from build123d import *

# Parameters (mm, degrees)
SKETCH1_R           = 22.5
BOSS_EXTRUDE1_DEPTH = 89
SKETCH2_R           = 21
BOSS_EXTRUDE2_DEPTH = 20
SKETCH3_R           = 16
BOSS_EXTRUDE3_DEPTH = 20
CHAMFER1_SIZE       = 5
SKETCH4_R           = 5
BOSS_EXTRUDE4_DEPTH = 13
SKETCH5_R           = 3
CUT_EXTRUDE1_DEPTH  = 10


with BuildPart() as part:
    # Sketch1 → Boss-Extrude1 (new body)
    with BuildSketch(Plane.XY):
        Circle(SKETCH1_R)
    extrude(amount=BOSS_EXTRUDE1_DEPTH)

    # Sketch2 → Boss-Extrude2 (add)
    with BuildSketch(Plane.XY.offset(89)):
        Circle(SKETCH2_R)
    extrude(amount=BOSS_EXTRUDE2_DEPTH)

    # Sketch3 → Boss-Extrude3 (add)
    with BuildSketch(Plane.XY.offset(109)):
        Circle(SKETCH3_R)
    extrude(amount=BOSS_EXTRUDE3_DEPTH)

    # Chamfer1
    chamfer1_edges = [part.edges().sort_by_distance(p)[0] for p in [
        (-16, 0, 129),
    ]]
    chamfer(chamfer1_edges, length=CHAMFER1_SIZE)

    # Sketch4 → Boss-Extrude4 (add)
    with BuildSketch(Plane.XY.offset(129)):
        with Locations(Location((0, 0, 0), (0, 0, 180))):
            Circle(SKETCH4_R)
    extrude(amount=BOSS_EXTRUDE4_DEPTH)

    # Sketch5 → Cut-Extrude1 (cut)
    with BuildSketch(Plane.XY.offset(142)):
        Circle(SKETCH5_R)
    extrude(amount=-CUT_EXTRUDE1_DEPTH, mode=Mode.SUBTRACT)


solid = part.part
The listing builds one solid part. Answer for the finished solid, in the listing's coordinates (mm). A direction names the side the tool comes from. Coordinates: 2 decimals unless noted, no trailing zeros. Order: outer loops, then holes, each group sorted by start corner. A loop starts at its lowest first (then second) coordinate and runs counter-clockwise, first axis right, second up.
Q1. For a pull along Y with two mould halves and no side action, classify faces 3 (the face through (-3, 0, 137)), 4 (the face through (0.1, 3.3, 142)), 5 (the face through (-8.9, -6.8, 128.8)) as pulls with the +Y half, pulls with the -Y half, needs draft (parallel to the pull), parting line crosses it, or undercut.
Q2. Given P1, Ø5, axis at x = 0.5, y = 10.5, coming from the +Z side; P2, Ø3, axis at x = 12.5, z = 27.5, coming from the -Y side; P3, Ø2, axis at x = -15.5, y = 3, coming from the +Z side, each flat-ended and moving along its own axis, determine where each tip first touches the part or whether it passes through.
Q3. A cutting plane is placed at D-D, the plane z = 116.5. Write down the section's boundary in (x, y), and give its area (3 significant figures).
Q4. Consider line 1 (Y direction, x = 0, z = 134.25); line 2 (Z direction, x = -8, y = -17.5); line 3 (Z direction, x = 9, y = -5). Determine where each line is inside the solid, lowest interval first.
Q5. A cutting plane is placed at C-C, the plane z = 9. Write down the section's boundary in (x, y), and give its area (3 significant figures).
Q6. A cutting plane is placed at A-A, the plane y = 0. Write down the section's boundary in (x, z).
Q7. Which of the six approach directions +Z, -Z, +X, -X, +Y, -Y give full straight-line access (tool end or side, diameter ignored) to faces 1 (the face through (-7, -20, 89)), 2 (the face through (0, 0, 0))?
Answers follow:
1. face 3: undercut
1. face 4: needs draft
1. face 5: parting line crosses it
2. P1: stops at z = 129
2. P2: stops at y = -19.63
2. P3: stops at z = 125.21
3. outline: circle Ø32 at (0, 0)
3. area: 804 mm2
4. line 1: y = -5 to -3, 3 to 5
4. line 2: z = 0 to 109
4. line 3: z = 0 to 129
5. outline: circle Ø45 at (0, 0)
5. area: 1,590 mm2
6. outline: (-22.5, 0) - (22.5, 0) - (22.5, 89) - (21, 89) - (21, 109) - (16, 109) - (16, 124) - (11, 129) - (5, 129) - (5, 142) - (3, 142) - (3, 132) - (-3, 132) - (-3, 142) - (-5, 142) - (-5, 129) - (-11, 129) - (-16, 124) - (-16, 109) - (-21, 109) - (-21, 89) - (-22.5, 89) - close
7. face 1: +Z
7. face 2: -Z, +X, -X, +Y, -Y
